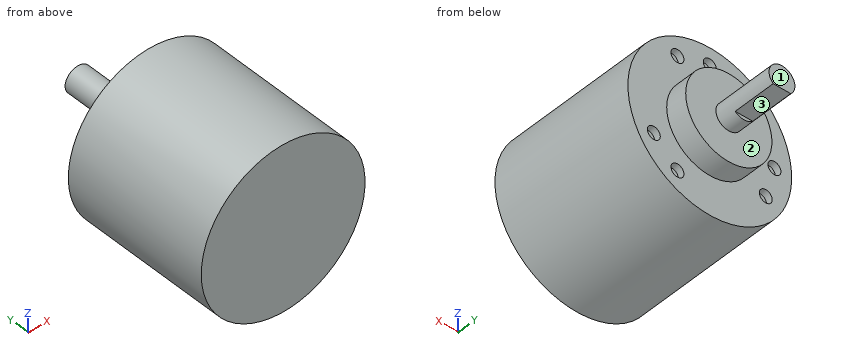
Autodesk Inventor part; units mm, degrees
ref_plane "YZ Plane" through (0, 0, 0) normal (1, 0, 0) x (0, 1, 0)
ref_plane "XZ Plane" through (0, 0, 0) normal (0, 1, 0) x (-1, 0, 0)
ref_plane "XY Plane" through (0, 0, 0) normal (0, 0, 1) x (1, 0, 0)
sketch "草图1" plane through (0, 0, 0) normal (0, 1, 0) x (-1, 0, 0)
  circle A0 centre (0, 0) radius 19
  circle A1 centre (0, 0) radius 10
  dimension "d0" = 38
  dimension "d1" = 20
extrude "拉伸1" add sketch "草图1" against normal blind 35 contours A0 | A1
sketch "草图2" plane through (0, 0, 0) normal (0, 1, 0) x (1, 0, 0)
  circle A0 centre (0, 0) radius 10
  circle A1 centre (0, 0) radius 15
  circle A2 centre (-15, 0) radius 1.5
  circle A3 centre (7.5, -12.9904) radius 1.5
  circle A4 centre (7.5, 12.9904) radius 1.5
  line L0 (0, 0) -> (-12.9904, 7.5)
  line L1 (0, 0) -> (15, 0) construction
  circle A5 centre (-12.9904, 7.5) radius 1.5
  circle A6 centre (0, -15) radius 1.5
  circle A7 centre (12.9904, 7.5) radius 1.5
  dimension "d4" = 20
  dimension "d5" = 30
  dimension "d6" = 3
  dimension "d9" = 360
  dimension "d11" = 150
  dimension "d12" = 3
  dimension "d15" = 360
extrude "拉伸2" cut sketch "草图2" against normal blind 1.5 contours A5 A1 L0 | L0 A1 A5 | A1 A5 | A2 A1 | A1 A2 | A4 A1 | A1 A4 | A6 A1 | A1 A6 | A7 A1 | A1 A7 | A3 A1 | A1 A3
sketch "草图3" plane through (0, 0, 0) normal (0, 1, 0) x (1, 0, 0)
  circle A0 centre (0, 0) radius 10
  dimension "d19" = 20
extrude "拉伸3" add sketch "草图3" along normal blind 5
sketch "草图4" plane through (0, 5, 0) normal (0, 1, 0) x (1, 0, 0)
  circle A0 centre (0, 0) radius 3
  dimension "d22" = 6
extrude "拉伸4" add sketch "草图4" along normal blind 14
sketch "草图5" plane through (0, 19, 0) normal (0, 1, 0) x (1, 0, 0)
  circle A0 centre (0, 0) radius 3
  line L0 (0, -3) -> (0, 2.2)
  line L1 (0, 2.2) -> (-2.0396, 2.2)
  line L2 (0, 2.2) -> (2.0396, 2.2)
  dimension "d25" = 5.2
extrude "拉伸5" cut sketch "草图5" against normal blind 10 contours L2 L1 A0
thread "螺纹1"
thread "螺纹2"
thread "螺纹3"
thread "螺纹4"
thread "螺纹5"
thread "螺纹6"
properties part number "rotary_encoder"
Source: CAD feature listing. Evaluate the final solid. Frame: model axes, mm. Face numbers are marked on the shaded views. A direction names the side the tool comes from. Round coordinates to 2 decimals unless told otherwise and drop trailing zeros. Loops run counter-clockwise (first coordinate to the right, second up) from the corner with the lowest first, then second, coordinate; pieces in that order, holes last. Notation, with made-up numbers: M 1,-32 L 18,-32 A22 ccw 18,-9 Z; hole C 40,65 d5. An arc over 180 degrees is marked long. Return JSON: item names as keys, results as strings. Group by question number.
1. Section query D-D on x = -8. Output: boundary loops of the cut face in (y, z), and give its area (3 significant figures).
2. Pin query (flat end, axial travel): pin 1 (1.2 mm diameter, centred on x = 0, y = 14, fed in from -Z); pin 2 (8 mm diameter, centred on y = -6.5, z = -12.5, fed in from +X); pin 3 (3.5 mm diameter, centred on x = 0.5, z = 15, fed in from +Y); pin 4 (19 mm diameter, centred on x = -8.5, z = -7.5, fed in from +Y). Return the tip coordinate at first contact, or that it passes through.
3. Reachability of the marked faces 1, 2 and 3 from +Z, -Z, +X, -X, +Y, -Y: full face, straight path, thin tool, end or side. Return the list, or none.
4. Section query A-A on x = 0. Output: boundary loops of the cut face in (y, z).
5. Material intervals for line 1 along X through (y, z) = (-0.65, -7.5); line 2 along Z through (x, y) = (7, -1), sorted ascending. Write a range as from..to.
6. Section query C-C on y = -19.5. Output: boundary loops of the cut face in (x, z).
7. Section query B-B on z = 0. Output: boundary loops of the cut face in (x, y), and give its area (3 significant figures).
Checks:
{
 "1": {"outline": "M -35,-17.23 L 0,-17.23 L 0,-6 L 5,-6 L 5,6 L 0,6 L 0,17.23 L -35,17.23 Z", "area": "1,270 mm²"},
 "2": {"pin 1": "stops at z = -2.2", "pin 2": "stops at x = 16.99", "pin 3": "stops at y = 0", "pin 4": "stops at y = 19"},
 "3": {"face 1": "+Z, -Z, +X, -X, +Y", "face 2": "+Y", "face 3": "-Z, +X, -X, +Y"},
 "4": {"outline": "M -35,-19 L 0,-19 L 0,-10 L 5,-10 L 5,-3 L 9,-3 L 9,-2.2 L 19,-2.2 L 19,3 L 5,3 L 5,10 L 0,10 L 0,13.5 L -1.5,13.5 L -1.5,16.5 L 0,16.5 L 0,19 L -35,19 Z"},
 "5": {"line 1": "x = -17.46..-14.49, -11.49..11.49, 14.49..17.46", "line 2": "z = -17.66..-14.4, -11.58..11.58, 14.4..17.66"},
 "6": {"outline": "C 0,0 d38"},
 "7": {"outline": "M -19,-35 L 19,-35 L 19,0 L 10,0 L 10,5 L 3,5 L 3,19 L -3,19 L -3,5 L -10,5 L -10,0 L -13.5,0 L -13.5,-1.5 L -16.5,-1.5 L -16.5,0 L -19,0 Z", "area": "1,510 mm²"}
}
